from build123d import *

# Parameters (mm, degrees)
SKETCH_1_W          = 20
SKETCH_1_H          = 20
EXTRUDE_1_DEPTH     = 3
EXTRUDE_2_DEPTH     = 3
EXTRUDE_3_DEPTH     = 3
SKETCH_6_R          = 1.6
CUT_EXTRUDE_1_DEPTH = 21
SKETCH_8_R          = 2
CUT_EXTRUDE_2_DEPTH = 4


with BuildPart() as part:
    # 草图1 → 凸台-拉伸1 (new body)
    with BuildSketch(Plane(origin=(0, 0, 0), x_dir=(1, 0, 0), z_dir=(0, 1, 0))):
        Rectangle(SKETCH_1_W, SKETCH_1_H)
    extrude(amount=EXTRUDE_1_DEPTH)

    # 草图4 → 凸台-拉伸2 (add)
    with BuildSketch(Plane.ZY.offset(10)):
        Polygon((10, 3), (10, 43), (0, 43), (-5, 3), align=None)
    extrude(amount=-EXTRUDE_2_DEPTH)

    # 草图5 → 凸台-拉伸3 (add)
    with BuildSketch(Plane(origin=(10, 0, 0), x_dir=(0, 0, -1), z_dir=(1, 0, 0))):
        Polygon((-10, 3), (5, 3), (0, 43), (-10, 43), align=None)
    extrude(amount=-EXTRUDE_3_DEPTH)

    # 草图6 → 切除-拉伸1 (cut, through all)
    with BuildSketch(Plane(origin=(10, 0, 0), x_dir=(0, 0, -1), z_dir=(1, 0, 0))):
        with Locations((-4.5, 38.5)):
            Circle(SKETCH_6_R)
    extrude(amount=-CUT_EXTRUDE_1_DEPTH, mode=Mode.SUBTRACT)

    # 草图8 → 切除-拉伸2 (cut, through all)
    with BuildSketch(Plane(origin=(0, 3, 0), x_dir=(1, 0, 0), z_dir=(0, 1, 0))):
        Circle(SKETCH_8_R)
    extrude(amount=-CUT_EXTRUDE_2_DEPTH, mode=Mode.SUBTRACT)


solid = part.part
Design review of the part built by this model. Coordinates are the model's own, in mm. A direction names the side the tool comes from. Give positions to 0.01 mm unless a question says otherwise; leave off trailing zeros. Order: outer loops, then holes, each group sorted by start corner. A loop starts at its lowest first (then second) coordinate and runs counter-clockwise, first axis right, second up. Notation, with made-up numbers: (83, 23.5) - (134, 23.5) arc R14 cw to (134, 42.5) - close; hole circle Ø4 at (70, -22). An arc over 180 degrees is marked (long way). Write item = value, one per line. Start each with the question number.
Q1. Mouldability with a two-part tool opening along Z and no side actions: class faces 3 (the face through (-8.521, 23.28, -2.465)), 4 (the face through (-9, 43, 5)), 5 (the face through (0, 2, 2)) as released by +Z, released by -Z, zero draft, split by the parting line, or undercut.
Q2. We need section B-B on x = 0. State the section outline as (y, z) points.
Q3. Clearance check with flat-ended pins moving along their axes: pin 1 Ø8 at (x, z) = (2.5, 3) entering from -Y; pin 2 Ø4 at (x, z) = (1.5, -2) entering from +Y. State where each tip first meets the part, or that it passes through.
Q4. To check wall thickness, follow L1, parallel to X at y = 7, z = 4.75; L2, parallel to X at y = 0.8, z = 0. State the ranges of each line that lie inside material, in increasing order. Write a range as from..to.
Q5. We need section C-C on y = 39. State the section outline as (x, z) points, plus the area to 3 significant figures.
Q6. We need section D-D on x = -7.75. State the section outline as (y, z) points.
Q7. We need section A-A on z = 4.5. State the section outline as (x, y) points.
Q8. Tool access review of faces 1 (the face through (7, 23, 4)), 2 (the face through (-8.48, 37.08, 3.76)): name each direction out of +Z, -Z, +X, -X, +Y, -Y from which nothing blocks a thin tool from reaching the whole face with its end or side.
Working result:
q1.face_3 = released by -Z
q1.face_4 = zero draft
q1.face_5 = undercut
q2.outline = (0, -10) - (3, -10) - (3, -2) - (0, -2) - close; (0, 2) - (3, 2) - (3, 10) - (0, 10) - close
q3.pin_1 = 0
q3.pin_2 = 3
q4.L1 = -10..-7, 7..10
q4.L2 = -10..-2, 2..10
q5.outline = (-10, -0.5) - (-7, -0.5) - (-7, 2.98) - (-10, 2.98) - close; (-10, 6.02) - (-7, 6.02) - (-7, 10) - (-10, 10) - close; (7, -0.5) - (10, -0.5) - (10, 2.98) - (7, 2.98) - close; (7, 6.02) - (10, 6.02) - (10, 10) - (7, 10) - close
q5.area = 44.8 mm²
q6.outline = (0, -10) - (3, -10) - (3, -5) - (43, 0) - (43, 10) - (0, 10) - close; hole circle Ø3.2 at (38.5, 4.5)
q7.outline = (-10, 0) - (10, 0) - (10, 36.9) - (7, 36.9) - (7, 3) - (-7, 3) - (-7, 36.9) - (-10, 36.9) - close; (-10, 40.1) - (-7, 40.1) - (-7, 43) - (-10, 43) - close; (7, 40.1) - (10, 40.1) - (10, 43) - (7, 43) - close
q8.face_1 = +Z, -Z, +Y
q8.face_2 = +X, -X
